Design review of the part built by this model. Coordinates are the model's own, in mm. A direction names the side the tool comes from. Round coordinates to 2 decimals unless told otherwise and drop trailing zeros. Order: outer loops, then holes, each group sorted by start corner. A loop starts at its lowest first (then second) coordinate and runs counter-clockwise, first axis right, second up. Notation, with made-up numbers: M 31,25.25 L 67,25.25 A15 cw 67,45.25 Z; hole C 84.5,63 d3. An arc over 180 degrees is marked long. Use a Markdown table: item, result. Add a question column.
(1) Take a section at B-B (y = 30). Write out the cut boundary in (x, z), then the cut area to 3 significant figures.
(2) Take a section at C-C (x = 24.5). Write out the cut boundary in (y, z), then the cut area to 3 significant figures.
(3) Take a section at A-A (x = 74.9). Write out the cut boundary in (y, z).
(4) To check wall thickness, follow probe 1 along X at (y, z) = (83, 0.7); probe 2 along Y at (x, z) = (75.5, 3.4); probe 3 along X at (y, z) = (70, 2.4). State the ranges of each line that lie inside material, in increasing order. Write a range as from..to.
(5) Machinability: for faces 1 (the face through (53.333, 113, 3)), 2 (the face through (39.667, 62.697, 2.465)), 3 (the face through (53.352, -3, 2)), which of the approach directions +Z, -Z, +X, -X, +Y, -Y give a long, thin tool a straight path to every point of the face, cutting with its end or side? Answer none if there is none.
(6) For pin 1 (3.5 mm diameter, centred on x = 74.9, y = 86.68, fed in from +Z); pin 2 (2.5 mm diameter, centred on y = 112.5, z = 1.5, fed in from +X); pin 3 (1.5 mm diameter, centred on y = -2, z = 3, fed in from -X) (3 decimals); pin 4 (1.5 mm diameter, centred on x = 19, z = 2.5, fed in from -Y), all flat-tipped, find the tip position at first contact; note any pin that passes through.
(7) The part is to be moulded in two halves that separate along Y. For faces 4 (the face through (26.685, -3, 2)), 5 (the face through (5.941, 53.654, 2.535)), 6 (the face through (13, 110.929, 2)), say which applies: released by +Y, released by -Y, zero draft, split by the parting line, or undercut.
(8) Take a section at D-D (z = 2.4). Count the separate pieces of the cut face and the enclosed holes in it, then the cut area to 3 significant figures.
```python
from build123d import *

# Parameters (mm, degrees)
CROQUIS1_W              = 79.981686337
CROQUIS1_H              = 111
SALIENTE_EXTRUIR1_DEPTH = 5
CROQUIS2_W              = 26.666666667
CROQUIS2_H              = 5
SALIENTE_EXTRUIR2_DEPTH = 5
CROQUIS3_W              = 26.666666666
CROQUIS3_H              = 5
SALIENTE_EXTRUIR3_DEPTH = 5
CROQUIS4_R              = 2
CORTAR_EXTRUIR1_DEPTH   = 10


with BuildPart() as part:
    # Croquis1 → Saliente-Extruir1 (new body)
    with BuildSketch(Plane.XY):
        with Locations((40.009156832, 55.428810295)):
            Rectangle(CROQUIS1_W, CROQUIS1_H)
        Polygon((40.989314194, 48.912995634), (38.382171337, 47.428810295), (59.160766092, 10.928810295), (61.767908949, 12.412995634), align=None, mode=Mode.SUBTRACT)
        Polygon((49.160766092, 10.928810295), (51.767908949, 12.412995634), (30.989314194, 48.912995634), (28.382171337, 47.428810295), align=None, mode=Mode.SUBTRACT)
        Polygon((20.989314194, 48.912995634), (18.382171337, 47.428810295), (39.160766092, 10.928810295), (41.767908949, 12.412995634), align=None, mode=Mode.SUBTRACT)
        Polygon((29.160766092, 10.928810295), (31.767908949, 12.412995634), (10.989314194, 48.912995634), (8.382171337, 47.428810295), align=None, mode=Mode.SUBTRACT)
        Polygon((38.382171337, 63.428810295), (40.989314194, 61.944624955), (61.767908949, 98.444624955), (59.160766092, 99.928810295), align=None, mode=Mode.SUBTRACT)
        Polygon((51.767908949, 98.444624955), (49.160766092, 99.928810295), (28.382171337, 63.428810295), (30.989314194, 61.944624955), align=None, mode=Mode.SUBTRACT)
        Polygon((18.382171337, 63.428810295), (20.989314194, 61.944624955), (41.767908949, 98.444624955), (39.160766092, 99.928810295), align=None, mode=Mode.SUBTRACT)
        Polygon((31.767908949, 98.444624955), (29.160766092, 99.928810295), (8.382171337, 63.428810295), (10.989314194, 61.944624955), align=None, mode=Mode.SUBTRACT)
    extrude(amount=SALIENTE_EXTRUIR1_DEPTH)

    # Croquis2 → Saliente-Extruir2 (add)
    with BuildSketch(Plane.XZ.offset(0.071189705)):
        with Locations((40.018313663, 2.5)):
            Rectangle(CROQUIS2_W, CROQUIS2_H)
    extrude(amount=SALIENTE_EXTRUIR2_DEPTH)

    # Croquis3 → Saliente-Extruir3 (add)
    with BuildSketch(Plane(origin=(0, 110.928810295, 0), x_dir=(1, 0, 0), z_dir=(0, 1, 0))):
        with Locations((40, -2.5)):
            Rectangle(CROQUIS3_W, CROQUIS3_H)
    extrude(amount=SALIENTE_EXTRUIR3_DEPTH)

    # Croquis4 → Cortar-Extruir1 (cut)
    with BuildSketch(Plane.XY.offset(5)):
        with Locations((74.9, 55.428810295)):
            Circle(CROQUIS4_R)
        with Locations((74.9, 86.678810295)):
            Circle(CROQUIS4_R)
        with Locations((74.9, 24.178810295)):
            Circle(CROQUIS4_R)
        with Locations((5.018313663, 55.428810295)):
            Circle(CROQUIS4_R)
        with Locations((5.018313663, 86.678810295)):
            Circle(CROQUIS4_R)
        with Locations((5.018313663, 24.178810295)):
            Circle(CROQUIS4_R)
    extrude(amount=-CORTAR_EXTRUIR1_DEPTH, mode=Mode.SUBTRACT)


solid = part.part
```
Verdict:
| question | item | result |
|---|---|---|
| 1 | outline | M 0.02,0 L 18.3,0 L 18.3,5 L 0.02,5 Z; M 21.76,0 L 28.3,0 L 28.3,5 L 21.76,5 Z; M 31.76,0 L 38.3,0 L 38.3,5 L 31.76,5 Z; M 41.76,0 L 48.3,0 L 48.3,5 L 41.76,5 Z; M 51.76,0 L 80,0 L 80,5 L 51.76,5 Z |
| 1 | area | 331 mm^2 |
| 2 | outline | M -0.07,0 L 19.12,0 L 19.12,5 L -0.07,5 Z; M 25.18,0 L 36.68,0 L 36.68,5 L 25.18,5 Z; M 42.75,0 L 68.11,0 L 68.11,5 L 42.75,5 Z; M 74.18,0 L 85.68,0 L 85.68,5 L 74.18,5 Z; M 91.74,0 L 110.93,0 L 110.93,5 L 91.74,5 Z |
| 2 | area | 434 mm^2 |
| 3 | outline | M -0.07,0 L 22.18,0 L 22.18,5 L -0.07,5 Z; M 26.18,0 L 53.43,0 L 53.43,5 L 26.18,5 Z; M 57.43,0 L 84.68,0 L 84.68,5 L 57.43,5 Z; M 88.68,0 L 110.93,0 L 110.93,5 L 88.68,5 Z |
| 4 | probe 1 | x = 0.02..19.52, 22.98..29.52, 32.98..39.52, 42.98..49.52, 52.98..80 |
| 4 | probe 2 | y = -0.07..22.27, 26.09..53.52, 57.34..84.77, 88.59..110.93 |
| 4 | probe 3 | x = 0.02..12.12, 15.58..22.12, 25.58..32.12, 35.58..42.12, 45.58..80 |
| 5 | face 1 | +Z, -Z, +X, +Y |
| 5 | face 2 | +Z, -Z |
| 5 | face 3 | +Z, -Z, +X, -Y |
| 6 | pin 1 | passes through |
| 6 | pin 2 | stops at x = 53.33 |
| 6 | pin 3 | stops at x = 26.685 |
| 6 | pin 4 | stops at y = -0.07 |
| 7 | face 4 | zero draft |
| 7 | face 5 | undercut |
| 7 | face 6 | released by +Y |
| 8 | separate pieces | 1 |
| 8 | enclosed holes | 14 |
| 8 | area | 8,060 mm^2 |
